from build123d import *

# Parameters (mm, degrees)
SKETCH1_R           = 3.96875
SKETCH1_R_2         = 2.55
SKETCH1_R_3         = 27.5336
BOSS_EXTRUDE7_DEPTH = 10
SKETCH2_W           = 73
SKETCH2_H           = 10.538321467
BOSS_EXTRUDE8_DEPTH = 30
FILLET3_R           = 20
FILLET4_R           = 20
CUT_EXTRUDE1_DEPTH  = 298.489495613
CUT_EXTRUDE2_DEPTH  = 298.489495613


with BuildPart() as part:
    # Sketch1 → Boss-Extrude7 (new body)
    with BuildSketch(Plane(origin=(0, 0, 0), x_dir=(1, 0, 0), z_dir=(0, 1, 0))):
        with BuildLine():
            Line((0, 70), (0, 0))
            Line((0, 0), (178.818297442, 0))
            ThreePointArc((178.818297442, 0), (164.66, 35), (178.818297442, 70))
            Line((178.818297442, 70), (0, 70))
        make_face()
        with Locations(Location((14, 35, 0), (0, 0, 270))):
            Circle(SKETCH1_R, mode=Mode.SUBTRACT)
        with Locations(Location((25.318924397, 35, 0), (0, 0, 270))):
            Circle(SKETCH1_R_2, mode=Mode.SUBTRACT)
        with Locations((58, 35)):
            Circle(SKETCH1_R_3, mode=Mode.SUBTRACT)
        with BuildLine():
            ThreePointArc((265.34, 35), (261.666382476, 16.122385039), (251.181702558, 0))
            Line((251.181702558, 0), (280, 0))
            Line((280, 0), (280, 70))
            Line((280, 70), (251.181702558, 70))
            ThreePointArc((251.181702558, 70), (261.666382476, 53.877614961), (265.34, 35))
        make_face()
        with Locations(Location((272.5, 35, 0), (0, 0, 270))):
            Circle(SKETCH1_R, mode=Mode.SUBTRACT)
        with Locations(Location((270, 59, 0), (0, 0, 270))):
            Circle(SKETCH1_R, mode=Mode.SUBTRACT)
        with BuildLine():
            ThreePointArc((178.818297442, 70), (164.66, 35), (178.818297442, 0))
            Line((178.818297442, 0), (251.181702558, 0))
            ThreePointArc((251.181702558, 0), (261.666382476, 16.122385039), (265.34, 35))
            ThreePointArc((265.34, 35), (261.666382476, 53.877614961), (251.181702558, 70))
            Line((251.181702558, 70), (178.818297442, 70))
        make_face()
        with Locations((215, 35)):
            Circle(SKETCH1_R_3, mode=Mode.SUBTRACT)
        with Locations((215, 35)):
            Circle(SKETCH1_R_3)
        with Locations(Location((215, 35, 0), (0, 0, 270))):
            Circle(SKETCH1_R, mode=Mode.SUBTRACT)
        with Locations((58, 35)):
            Circle(SKETCH1_R_3)
        with Locations(Location((58, 35, 0), (0, 0, 270))):
            Circle(SKETCH1_R, mode=Mode.SUBTRACT)
    extrude(amount=BOSS_EXTRUDE7_DEPTH)

    # Sketch2 → Boss-Extrude8 (add)
    with BuildSketch(Plane(origin=(0, 0, -70), x_dir=(-1, 0, 0), z_dir=(0, 0, -1))):
        with Locations((-148.5, 5.269160734)):
            Rectangle(SKETCH2_W, SKETCH2_H)
    extrude(amount=BOSS_EXTRUDE8_DEPTH)

    # Fillet3
    fillet3_edges = [part.edges().sort_by_distance(p)[0] for p in [
        (185, 5.269160734, -100),
    ]]
    fillet(fillet3_edges, radius=FILLET3_R)

    # Fillet4
    fillet4_edges = [part.edges().sort_by_distance(p)[0] for p in [
        (112, 5.269160734, -100),
    ]]
    fillet(fillet4_edges, radius=FILLET4_R)

    # Sketch3 → Cut-Extrude1 (cut, through all)
    with BuildSketch(Plane(origin=(0, 10, 0), x_dir=(1, 0, 0), z_dir=(0, 1, 0))):
        with BuildLine():
            Line((121, 61.05), (121, 66.13))
            ThreePointArc((121, 66.13), (105.392513422, 60.402805839), (97.193821375, 45.939893305))
            Line((97.193821375, 45.939893305), (102.361874001, 45.939893305))
            ThreePointArc((102.361874001, 45.939893305), (109.003176826, 56.797930049), (121, 61.05))
        make_face()
    extrude(amount=-CUT_EXTRUDE1_DEPTH, mode=Mode.SUBTRACT)

    # Sketch3_3 → Cut-Extrude2 (cut, through all)
    with BuildSketch(Plane(origin=(0, 10, 0), x_dir=(1, 0, 0), z_dir=(0, 1, 0))):
        with BuildLine():
            Line((121, 17.87), (121, 22.95))
            ThreePointArc((121, 22.95), (109.003176826, 27.202069951), (102.361874001, 38.060106695))
            Line((102.361874001, 38.060106695), (97.193821375, 38.060106695))
            ThreePointArc((97.193821375, 38.060106695), (105.392513422, 23.597194161), (121, 17.87))
        make_face()
    extrude(amount=-CUT_EXTRUDE2_DEPTH, mode=Mode.SUBTRACT)


solid = part.part
Part model, mm, in its own coordinate system. A direction names the side the tool comes from. Round coordinates to 2 decimals unless told otherwise and drop trailing zeros. Write each loop counter-clockwise with the first axis right and the second up, starting at its lowest first coordinate (ties: lowest second). Pieces come first, ordered by that corner, then holes. Notation, with made-up numbers: M 1,-34 L 6,-34 A7 ccw 6,-29 Z; hole C 12,29.25 d7. An arc over 180 degrees is marked long. Return JSON: item names as keys, results as strings. Group by question number.
(1) Pin check, flat tips, straight feed: pin 1 Ø5.5 at (x, y) = (99.5, 2.5) entering from -Z; pin 2 Ø5 at (x, y) = (31.5, 6) entering from +Z; pin 3 Ø21 at (x, z) = (149, -20.5) entering from +Y; pin 4 Ø3 at (y, z) = (6.5, -74.5) entering from -X. Stop position of each tip, or through.
(2) Drill centre lines: probe 1 along X at (y, z) = (4, -59.5); probe 2 along Z at (x, y) = (270, 3.25); probe 3 along Z at (x, y) = (107, 3.25). Where is each one in solid material? Low to high.
(3) Saw through at B-B on z = -35. Write the cut outline in (x, y), then the cut area to 3 significant figures.
(4) Two-plate mould, pull along Z, no slides. Class faces 5 (the face through (142, 0, -38)), 6 (the face through (118.014, 5.343, -94.297)), 7 (the face through (105.212, 5.07, -23.752)), 8 (the face through (138, 5, 0)): +Z half, -Z half, draft (parallel to the pull), parting line (faces both ways), or undercut.
(5) Saw through at C-C on y = 6. Count the separate pieces of the cut face and the enclosed holes in it, then the cut area to 3 significant figures.
(6) Saw through at D-D on x = 254. Write the cut outline in (y, z).
(7) Which spindle directions (+Z, -Z, +X, -X, +Y, -Y) get a long thin tool onto all of the face, cutting with end or side? Do faces 1 (the face through (57, 5, -70)), 2 (the face through (233, 5, -70)), 3 (the face through (108.86, 5.07, -56.68)), 4 (the face through (149, 5, -100)). Say none if no direction does.
(8) Saw through at A-A on x = 14. Write the cut outline in (y, z).
Returned:
{
 "1": {"pin 1": "z = -70", "pin 2": "z = 0", "pin 3": "y = 10", "pin 4": "x = 112"},
 "2": {"probe 1": "0 to 104.39, 113.47 to 266.06, 273.94 to 280", "probe 2": "-70 to -62.97, -55.03 to -38.08, -31.92 to 0", "probe 3": "-70 to -61.65, -54.92 to -29.08, -22.35 to 0"},
 "3": {"outline": "M 0,0 L 10.03,0 L 10.03,10 L 0,10 Z; M 17.97,0 L 22.77,0 L 22.77,10 L 17.97,10 Z; M 27.87,0 L 54.03,0 L 54.03,10 L 27.87,10 Z; M 61.97,0 L 97.91,0 L 97.91,10 L 61.97,10 Z; M 103.28,0 L 211.03,0 L 211.03,10 L 103.28,10 Z; M 218.97,0 L 268.53,0 L 268.53,10 L 218.97,10 Z; M 276.47,0 L 280,0 L 280,10 L 276.47,10 Z", "area": "2,380 mm²"},
 "4": {"face 5": "draft", "face 6": "-Z half", "face 7": "undercut", "face 8": "+Z half"},
 "5": {"separate pieces": "1", "enclosed holes": "8", "area": "21,000 mm²"},
 "6": {"outline": "M 0,-70 L 10,-70 L 10,0 L 0,0 Z"},
 "7": {"face 1": "-Z, -X, +Y, -Y", "face 2": "-Z, +X, +Y, -Y", "face 3": "+Y, -Y", "face 4": "-Z, +X, -X, +Y, -Y"},
 "8": {"outline": "M 0,-70 L 10,-70 L 10,-38.97 L 0,-38.97 Z; M 0,-31.03 L 10,-31.03 L 10,0 L 0,0 Z"}
}
